```python
from build123d import *

# Parameters (mm, degrees)
SKETCH_1_W          = 36
SKETCH_1_H          = 38
EXTRUDE_1_DEPTH     = 2
CUT_EXTRUDE_1_REACH = 28.249
SKETCH_2_W          = 4
SKETCH_2_H          = 14
SKETCH_2_W_2        = 4.5
SKETCH_2_H_2        = 10.5
SKETCH_2_3_W        = 1.5
SKETCH_2_3_H        = 14
EXTRUDE_2_DEPTH     = 12
EXTRUDE_3_DEPTH     = 14
SKETCH_4_W          = 15
SKETCH_4_H          = 1
SKETCH_4_W_2        = 6
EXTRUDE_4_DEPTH     = 3
CUT_EXTRUDE_2_REACH = 30.792
SKETCH_5_W          = 5
SKETCH_5_H          = 4
SKETCH_6_R          = 0.75
EXTRUDE_5_DEPTH     = 2
SKETCH_7_R          = 2
EXTRUDE_6_DEPTH     = 2
EXTRUDE_7_DEPTH     = 2
FILLET_1_R          = 8
FILLET_2_R          = 1


with BuildPart() as part:
    # Sketch 1 → Extrude 1 (new body)
    with BuildSketch(Plane.XY):
        Rectangle(SKETCH_1_W, SKETCH_1_H)
    extrude(amount=EXTRUDE_1_DEPTH)

    # Sketch 2 → Cut-Extrude 1 (cut, up to next)
    with BuildSketch(Plane.XY.offset(2), mode=Mode.PRIVATE) as cut_extrude_1_sk1:
        with Locations((13.5, -2)):
            Rectangle(SKETCH_2_W, SKETCH_2_H)
    cut_extrude_1_tool1 = extrude(cut_extrude_1_sk1.sketch, amount=-CUT_EXTRUDE_1_REACH, mode=Mode.PRIVATE) & part.part
    # Sketch 2 → Cut-Extrude 1 (cut, up to next)
    with BuildSketch(Plane.XY.offset(2), mode=Mode.PRIVATE) as cut_extrude_1_sk2:
        with Locations((15.75, 13.75)):
            Rectangle(SKETCH_2_W_2, SKETCH_2_H_2)
    cut_extrude_1_tool2 = extrude(cut_extrude_1_sk2.sketch, amount=-CUT_EXTRUDE_1_REACH, mode=Mode.PRIVATE) & part.part
    cut_extrude_1_1 = cut_extrude_1_tool1.solids().sort_by_distance((13.5, -2, 2))[0]
    add(cut_extrude_1_1, mode=Mode.SUBTRACT)
    cut_extrude_1_2 = cut_extrude_1_tool2.solids().sort_by_distance((15.75, 13.75, 2))[0]
    add(cut_extrude_1_2, mode=Mode.SUBTRACT)
    cut_extrude_1 = cut_extrude_1_1 + cut_extrude_1_2  # Cut-Extrude 1 as one shape, for the pattern or mirror that repeats it

    # Sketch 2_3 → Extrude 2 (add)
    with BuildSketch(Plane.XY.offset(2)):
        with Locations((16.25, -2)):
            Rectangle(SKETCH_2_3_W, SKETCH_2_3_H)
    extrude_2 = extrude(amount=EXTRUDE_2_DEPTH)

    # Sketch 3 → Extrude 3 (add)
    with BuildSketch(Plane(origin=(0, 5, 0), x_dir=(1, 0, 0), z_dir=(0, 1, 0))):
        Polygon((15.5, -14), (14.5, -13), (15.5, -13), align=None)
    extrude_3 = extrude(amount=-EXTRUDE_3_DEPTH)

    # Mirror 1: Cut-Extrude 1, Extrude 2, Extrude 3 across plane
    add(cut_extrude_1.mirror(Plane(origin=(0, 0, 0), x_dir=(0, 0, 1), z_dir=(1, 0, 0))), mode=Mode.SUBTRACT)
    add(extrude_2.mirror(Plane(origin=(0, 0, 0), x_dir=(0, 0, 1), z_dir=(1, 0, 0))))
    add(extrude_3.mirror(Plane(origin=(0, 0, 0), x_dir=(0, 0, 1), z_dir=(1, 0, 0))))

    # Sketch 4 → Extrude 4 (add)
    with BuildSketch(Plane.XY.offset(2)):
        with Locations((0, -17)):
            Rectangle(SKETCH_4_W, SKETCH_4_H)
        with Locations((4.5, 13)):
            Rectangle(SKETCH_4_W_2, SKETCH_4_H)
    extrude(amount=EXTRUDE_4_DEPTH)

    # Sketch 5 → Cut-Extrude 2 (cut, up to next)
    with BuildSketch(Plane.XY.offset(2), mode=Mode.PRIVATE) as cut_extrude_2_sk1:
        with Locations((-8, 17)):
            Rectangle(SKETCH_5_W, SKETCH_5_H)
    cut_extrude_2_tool1 = extrude(cut_extrude_2_sk1.sketch, amount=-CUT_EXTRUDE_2_REACH, mode=Mode.PRIVATE) & part.part
    add(cut_extrude_2_tool1.solids().sort_by_distance((-8, 17, 2))[0], mode=Mode.SUBTRACT)

    # Sketch 6 → Extrude 5 (add)
    # profile 1 of 2: a face of its own
    with BuildSketch(Plane(origin=(3.5, 0, 0), x_dir=(0, 0, -1), z_dir=(1, 0, 0))):
        with BuildLine():
            Line((2.5, 21), (0, 19))
            Line((0, 19), (0, 17))
            Line((0, 17), (6.25, 17))
            ThreePointArc((6.25, 17), (8.25, 19), (6.25, 21))
            Line((6.25, 21), (2.5, 21))
        make_face()
        with Locations((6.25, 19)):
            Circle(SKETCH_6_R, mode=Mode.SUBTRACT)
    # profile 2 of 2: a face of its own
    with BuildSketch(Plane(origin=(3.5, 0, 0), x_dir=(0, 0, -1), z_dir=(1, 0, 0))):
        with BuildLine():
            ThreePointArc((7.423710101, -10.619384019), (8.152467876, -8.383059175), (6.25, -7))
            Line((6.25, -7), (0, -7))
            Line((0, -7), (0, -16))
            Line((0, -16), (7.423710101, -10.619384019))
        make_face()
        with Locations(Location((6.25, -9, 0), (0, 0, 180))):
            Circle(SKETCH_6_R, mode=Mode.SUBTRACT)
    extrude(amount=-EXTRUDE_5_DEPTH)

    # Sketch 7 → Extrude 6 (add)
    with BuildSketch(Plane.ZY.offset(18)):
        with BuildLine():
            Line((0, -6.119622458), (0, 8.5))
            Line((0, 8.5), (-2.902017955, 12.938839014))
            ThreePointArc((-2.902017955, 12.938839014), (-8.438839014, 14.097982045), (-9.597982045, 8.561160986))
            Line((-9.597982045, 8.561160986), (0, -6.119622458))
        make_face()
        with Locations(Location((-6.25, 10.75, 0), (0, 0, 270))):
            Circle(SKETCH_7_R, mode=Mode.SUBTRACT)
    extrude(amount=-EXTRUDE_6_DEPTH)

    # Sketch 8 → Extrude 7 (add)
    with BuildSketch(Plane(origin=(0, 15, 0), x_dir=(1, 0, 0), z_dir=(0, 1, 0))):
        Polygon((-10.5, 0), (-12.5, 0), (-11.09431212, 4), (-9.09431212, 4), align=None)
        Polygon((-4.90568788, 4), (-6.90568788, 4), (-5.5, 0), (-3.5, 0), align=None)
    extrude(amount=EXTRUDE_7_DEPTH)

    # Fillet 1
    fillet_1_edges = [part.edges().sort_by_distance(p)[0] for p in [
        (18, -19, 1),
        (-18, -19, 1),
    ]]
    fillet(fillet_1_edges, radius=FILLET_1_R)

    # Fillet 2
    # the kernel refuses this fillet: 1 mm, written as the material it adds along each edge
    with BuildSketch(Plane(origin=(-13.5, 8.5, 2), x_dir=(-1, 0, 0), z_dir=(0, 0, -1)), Plane(origin=(-10.5, 15, 2), x_dir=(0, 1, 0), z_dir=(0, 0, -1)), Plane(origin=(-5.5, 15, 2), x_dir=(-1, 0, 0), z_dir=(0, 0, -1))) as fillet_2_piece_1:
        with BuildLine():
            CenterArc((FILLET_2_R, FILLET_2_R), FILLET_2_R, 180, 90)
            Line((0, FILLET_2_R), (0, 0))
            Line((0, 0), (FILLET_2_R, 0))
        make_face()
    extrude(amount=2)
    with BuildSketch(Plane(origin=(-12.5, 15, 0), x_dir=(-1, 0, 0), z_dir=(0, 1, 0))) as fillet_2_piece_2:
        with BuildLine():
            CenterArc((FILLET_2_R * 0.708529633191, -FILLET_2_R), FILLET_2_R, 90, 70.63740436)
            Line((-FILLET_2_R * 0.234909668247, -FILLET_2_R * 0.668454702186), (0, 0))
            Line((0, 0), (FILLET_2_R * 0.708529633191, 0))
        make_face()
    extrude(amount=2)
    with BuildSketch(Plane(origin=(-3.5, 15, 0), x_dir=(1, 0, 0), z_dir=(0, 1, 0))) as fillet_2_piece_3:
        with BuildLine():
            CenterArc((FILLET_2_R * 0.708529633191, FILLET_2_R), FILLET_2_R, 199.36259564, 70.63740436)
            Line((-FILLET_2_R * 0.234909668247, FILLET_2_R * 0.668454702186), (0, 0))
            Line((0, 0), (FILLET_2_R * 0.708529633191, 0))
        make_face()
    extrude(amount=2)
    with BuildSketch(Plane(origin=(13.5, 8.5, 2), x_dir=(1, 0, 0), z_dir=(0, 0, -1))) as fillet_2_piece_4:
        with BuildLine():
            CenterArc((FILLET_2_R, -FILLET_2_R), FILLET_2_R, 90, 90)
            Line((0, -FILLET_2_R), (0, 0))
            Line((0, 0), (FILLET_2_R, 0))
        make_face()
    extrude(amount=2)
    # the kernel refuses this fillet: 1 mm, written as the material it takes off along each edge
    with BuildSketch(Plane(origin=(19.5, -9, 14), x_dir=(0, 1, 0), z_dir=(-1, 0, 0)), Plane(origin=(13, 5, 14), x_dir=(0, -1, 0), z_dir=(1, 0, 0)), Plane(origin=(-19.5, -9, 14), x_dir=(0, 0, -1), z_dir=(1, 0, 0))) as fillet_2_2_piece_1:
        with BuildLine():
            CenterArc((FILLET_2_R, FILLET_2_R), FILLET_2_R, 180, 90)
            Line((0, FILLET_2_R), (0, 0))
            Line((0, 0), (FILLET_2_R, 0))
        make_face()
    extrude(amount=6.5, mode=Mode.SUBTRACT)
    with BuildSketch(Plane(origin=(-13, 5, 14), x_dir=(0, -1, 0), z_dir=(-1, 0, 0))) as fillet_2_2_piece_2:
        with BuildLine():
            CenterArc((FILLET_2_R, -FILLET_2_R), FILLET_2_R, 90, 90)
            Line((0, -FILLET_2_R), (0, 0))
            Line((0, 0), (FILLET_2_R, 0))
        make_face()
    extrude(amount=6.5, mode=Mode.SUBTRACT)
    with BuildSketch(Plane(origin=(-7.5, -20, 5), x_dir=(1, 0, 0), z_dir=(0, 1, 0)), Plane(origin=(1.5, 16, 5), x_dir=(0, 0, -1), z_dir=(0, -1, 0))) as fillet_2_2_piece_3:
        with BuildLine():
            CenterArc((FILLET_2_R, FILLET_2_R), FILLET_2_R, 180, 90)
            Line((0, FILLET_2_R), (0, 0))
            Line((0, 0), (FILLET_2_R, 0))
        make_face()
    extrude(amount=6, mode=Mode.SUBTRACT)
    with BuildSketch(Plane(origin=(7.5, -14, 5), x_dir=(0, 0, -1), z_dir=(0, -1, 0)), Plane(origin=(7.5, 10, 5), x_dir=(-1, 0, 0), z_dir=(0, 1, 0))) as fillet_2_2_piece_4:
        with BuildLine():
            CenterArc((FILLET_2_R, -FILLET_2_R), FILLET_2_R, 90, 90)
            Line((0, -FILLET_2_R), (0, 0))
            Line((0, 0), (FILLET_2_R, 0))
        make_face()
    extrude(amount=6, mode=Mode.SUBTRACT)
    with BuildSketch(Plane(origin=(-13.5, 19, 4.5), x_dir=(1, 0, 0), z_dir=(0, 0, -1)), Plane(origin=(-10.5, 19, 4.5), x_dir=(0, -1, 0), z_dir=(0, 0, -1)), Plane(origin=(-5.5, 19, 4.5), x_dir=(1, 0, 0), z_dir=(0, 0, -1)), Plane(origin=(18, 8.5, 4.5), x_dir=(0, -1, 0), z_dir=(0, 0, -1)), Plane(origin=(13.5, 19, 4.5), x_dir=(0, -1, 0), z_dir=(0, 0, -1))) as fillet_2_2_piece_5:
        with BuildLine():
            CenterArc((FILLET_2_R, FILLET_2_R), FILLET_2_R, 180, 90)
            Line((0, FILLET_2_R), (0, 0))
            Line((0, 0), (FILLET_2_R, 0))
        make_face()
    extrude(amount=7, mode=Mode.SUBTRACT)
    with BuildSketch(Plane(origin=(-4.90568788, 13.228675917, -4), x_dir=(0.33154529781413966, 0, 0.9434393014377414), z_dir=(0, 1, 0)), Plane(origin=(-11.09431212, 13.228675917, -4), x_dir=(1, 0, 0), z_dir=(0, 1, 0))) as fillet_2_2_piece_6:
        with BuildLine():
            CenterArc((FILLET_2_R * 0.708529633191, -FILLET_2_R), FILLET_2_R, 90, 70.63740436)
            Line((-FILLET_2_R * 0.234909668247, -FILLET_2_R * 0.668454702186), (0, 0))
            Line((0, 0), (FILLET_2_R * 0.708529633191, 0))
        make_face()
    extrude(amount=5.542648166, mode=Mode.SUBTRACT)
    with BuildSketch(Plane(origin=(-9.09431212, 11.471566067, -4), x_dir=(-0.33154529781413894, 0, 0.9434393014377417), z_dir=(0, 1, 0)), Plane(origin=(-6.90568788, 11.471566067, -4), x_dir=(1, 0, 0), z_dir=(0, 1, 0))) as fillet_2_2_piece_7:
        with BuildLine():
            CenterArc((FILLET_2_R * 1.41137357304, -FILLET_2_R), FILLET_2_R, 90, 109.36259564)
            Line((FILLET_2_R * 0.4679342716, -FILLET_2_R * 1.33154529781), (0, 0))
            Line((0, 0), (FILLET_2_R * 1.41137357304, 0))
        make_face()
    extrude(amount=9.056867865, mode=Mode.SUBTRACT)
    with BuildSketch(Plane(origin=(4.376952648, 21, -2.5), x_dir=(0, -0.6246950475544217, 0.7808688094430323), z_dir=(-1, 0, 0))) as fillet_2_2_piece_8:
        with BuildLine():
            CenterArc((FILLET_2_R * 0.350781059358, -FILLET_2_R), FILLET_2_R, 90, 38.659808254)
            Line((-FILLET_2_R * 0.273913988196, -FILLET_2_R * 0.219131190557), (0, 0))
            Line((0, 0), (FILLET_2_R * 0.350781059358, 0))
        make_face()
    extrude(amount=3.753905297, mode=Mode.SUBTRACT)


solid = part.part
```
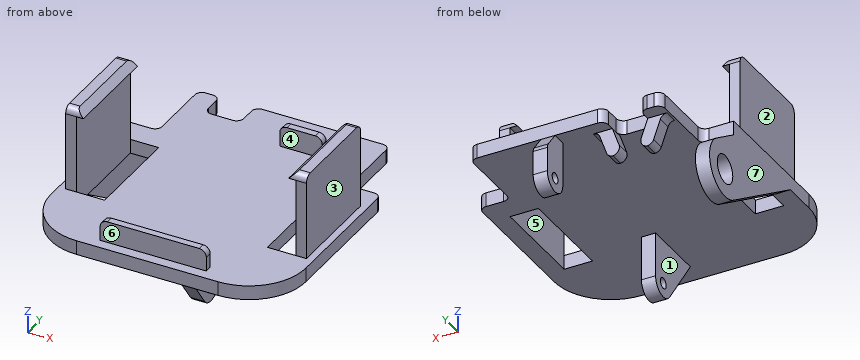
Read the model definition and answer for the solid it produces. Units are mm, in the model's axes. Face numbers are marked on the shaded views. A direction names the side the tool comes from. Round coordinates to 2 decimals unless told otherwise and drop trailing zeros. Write each loop counter-clockwise with the first axis right and the second up, starting at its lowest first coordinate (ties: lowest second). Pieces come first, ordered by that corner, then holes. Notation, with made-up numbers: M 35,37 L 71,37 A37 cw 71,76 Z; hole C 3,30.5 d10. An arc over 180 degrees is marked long. One line per item, written item: value.
Q1. Find section C-C on x = -2. Write down the section's boundary in (y, z).
Data:
outline: M -19,0 L 19,0 L 19,2 L -16.5,2 L -16.5,5 L -17.5,5 L -17.5,2 L -19,2 Z
Q2. Find section D-D on x = 14. Write down the section's boundary in (y, z), plus the area to 3 significant figures.
Data:
outline: M -17.93,0 L -9,0 L -9,2 L -17.93,2 Z; M 5,0 L 8.63,0 L 8.63,2 L 5,2 Z
area: 25.1 mm2
Q3. For a pull along X with two mould halves and no side action, classify the marked faces 5, 6 and 7 as +X half, -X half, draft (parallel to the pull), parting line (faces both ways), or undercut.
Data:
face 5: undercut
face 6: draft
face 7: -X half
Q4. Which of the six approach directions +Z, -Z, +X, -X, +Y, -Y give full straight-line access (tool end or side, diameter ignored) to the marked faces 1, 2, 3 and 4?
Data:
face 1: -Z, -X, +Y, -Y
face 2: +Z, -X, +Y, -Y
face 3: +Z, +X, +Y, -Y
face 4: +Z, +X, -X
Q5. Find section B-B on y = -4. Write down the section's boundary in (x, z).
Data:
outline: M -18,-1.39 L -16,-1.39 L -16,0 L -15.5,0 L -15.5,13 L -14.5,13 L -15.5,14 L -17,14 L -17,2 L -18,2 Z; M -11.5,0 L 11.5,0 L 11.5,2 L -11.5,2 Z; M 14.5,13 L 15.5,13 L 15.5,0 L 18,0 L 18,2 L 17,2 L 17,14 L 15.5,14 Z
Q6. Straight lines are drawn through the part: line 1 (X direction, y = 3.5, z = 10.5); line 2 (Z direction, x = 2.1, y = -9); line 3 (Y direction, x = 2.3, z = -6.25). For each, find the intervals that lie inside material, in ascending order. Write a range as [from, to].
Data:
line 1: [-17, -15.5], [15.5, 17]
line 2: [-8.25, -7], [-5.5, 2]
line 3: [-11.47, -9.75], [-8.25, -7], [17, 18.25], [19.75, 21]
Q7. Find section A-A on z = 3.5. Write down the section's boundary in (x, y).
Data:
outline: M -17,-9 L -15.5,-9 L -15.5,5 L -17,5 Z; M -7.5,-17.5 L 7.5,-17.5 L 7.5,-16.5 L -7.5,-16.5 Z; M 1.5,12.5 L 7.5,12.5 L 7.5,13.5 L 1.5,13.5 Z; M 15.5,-9 L 17,-9 L 17,5 L 15.5,5 Z
Q8. Flat-ended cylindrical pins translate along their axes: pin 1 Ø6 at (y, z) = (-8.5, 2.5) entering from -X; pin 2 Ø0.6 at (x, z) = (14, 1.5) entering from +Y; pin 3 Ø1.6 at (x, z) = (-16, 1.5) entering from +Y; pin 4 Ø1.1 at (x, z) = (-11.5, -2) entering from -Y. Find the tip coordinate at first contact, or state that the pin passes through.
Data:
pin 1: x = -18
pin 2: y = 8.9
pin 3: y = 8.5
pin 4: y = 15
